The listing builds one solid part. Answer for the finished solid, in the listing's coordinates (mm). Face numbers are marked on the shaded views. A direction names the side the tool comes from. Round coordinates to 2 decimals unless told otherwise and drop trailing zeros. Loops run counter-clockwise (first coordinate to the right, second up) from the corner with the lowest first, then second, coordinate; pieces in that order, holes last. Notation, with made-up numbers: (5, 11.25) - (18, 11.25) arc R31 ccw to (18, 41.25) - close; hole circle Ø11 at (20, 39.5). An arc over 180 degrees is marked (long way). Write item = value, one per line. Start each with the question number.
1) For a pull along Z with two mould halves and no side action, classify the marked faces 1, 2 and 3 as released by +Z, released by -Z, zero draft, split by the parting line, or undercut.
2) Section C-C, the plane y = -14 is taken. Determine the outline of the cut face in (x, z).
3) Section A-A, the plane z = -18.5 is taken. Determine the outline of the cut face in (x, y), and give its area (3 significant figures).
4) Straight lines are drawn through the part: line 1 along X through (y, z) = (-11.5, 36.5); line 2 along Y through (x, z) = (30, 21); line 3 along Z through (x, y) = (-33, 67). For each, find the intervals that lie inside material, in ascending order.
5) Section B-B, the plane x = 20.5 is taken. Determine the outline of the cut face in (y, z).
6) Given pin 1 Ø12.5 at (x, y) = (41.5, -8.5) entering from -Z; pin 2 Ø7.5 at (y, z) = (-9.5, 0.5) entering from -X; pin 3 Ø3 at (x, y) = (-37.5, -51.5) entering from +Z; pin 4 Ø4 at (x, z) = (5, 34) entering from +Y, each flat-ended and moving along its own axis, determine where each tip first touches the part or whether it passes through.
7) A tool of negligible diameter and unlimited length cuts with its end or side. For the marked faces 4, 5 and 6, from which of +Z, -Z, +X, -X, +Y, -Y can it reach the whole face along a straight path? Write none if from no direction.
8) Section D-D, the plane z = 33 is taken. Determine the outline of the cut face in (x, y).
from build123d import *

# Parameters (mm, degrees)
F1_DEPTH      = 25.4
F2_R          = 10.3575918664
F3_DEPTH      = 82.7624946833
F3_DEPTH_BACK = 25.4
F4_DEPTH      = 25.4
F5_DEPTH      = 211.4430963993


with BuildPart() as f1:
    # F0 (on Front) → F1 (new body)
    with BuildSketch(Plane.XZ):
        Polygon((-54.8551306129, 59.1857582331), (-54.8551306129, 13.9228226617), (-29.6127572656, 0), (-29.6127572656, -32.6884873211), (-54.8551306129, -32.6884873211), (-54.8551306129, -56.3453622162), (-17.4506641924, -56.3453622162), (-17.4506641924, 45.9188297391), (8.5172532126, 45.9188297391), (8.5172532126, 16.1184109747), (38.0811914802, 16.1184109747), (38.0811914802, -25.0818282366), (12.4506652355, -25.0818282366), (12.4506652355, -55.7573884726), (52.5093525648, -55.7573884726), (52.5093525648, 59.1857582331), align=None)
    extrude(amount=F1_DEPTH)

    # F2 (on Front) → F3 (join, two sides)
    with BuildSketch(Plane.XZ) as f3_sk:
        with Locations((-28.0219614506, 29.9158245325)):
            Circle(F2_R)
    extrude(amount=-F3_DEPTH)
    extrude(f3_sk.sketch, amount=F3_DEPTH_BACK)

    # F4 (add): a face of the model
    f4_faces = [f1.faces().sort_by_distance(p)[0] for p in [
        (-28.0219614506, 82.7624946833, 29.9158245325),
    ]]
    extrude(f4_faces, amount=F4_DEPTH)

    # F5 (add): a face of the model
    f5_faces = [f1.faces().sort_by_distance(p)[0] for p in [
        (-28.0219614506, 108.1624946833, 29.9158245325),
    ]]
    extrude(f5_faces, amount=-F5_DEPTH)


solid = f1.part
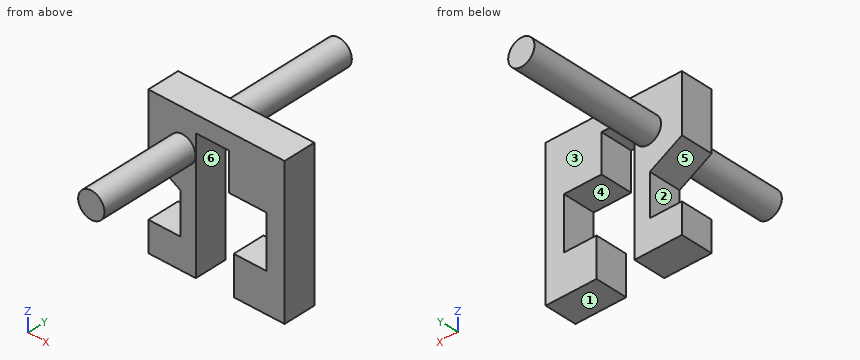
Geometry check:
q1.face_1 = released by -Z
q1.face_2 = undercut
q1.face_3 = zero draft
q2.outline = (-54.86, -56.35) - (-17.45, -56.35) - (-17.45, 45.92) - (8.52, 45.92) - (8.52, 16.12) - (38.08, 16.12) - (38.08, -25.08) - (12.45, -25.08) - (12.45, -55.76) - (52.51, -55.76) - (52.51, 59.19) - (-54.86, 59.19) - (-54.86, 13.92) - (-29.61, 0) - (-29.61, -32.69) - (-54.86, -32.69) - close
q3.outline = (-29.61, -25.4) - (-17.45, -25.4) - (-17.45, 0) - (-29.61, 0) - close; (38.08, -25.4) - (52.51, -25.4) - (52.51, 0) - (38.08, 0) - close
q3.area = 675 mm2
q4.line_1 = -54.86 to -17.45, 8.52 to 52.51
q4.line_2 = -25.4 to 0
q4.line_3 = 20.83 to 39
q5.outline = (-25.4, -55.76) - (0, -55.76) - (0, -25.08) - (-25.4, -25.08) - close; (-25.4, 16.12) - (0, 16.12) - (0, 59.19) - (-25.4, 59.19) - close
q6.pin_1 = -55.76
q6.pin_2 = -37.32
q6.pin_3 = 36.52
q6.pin_4 = through
q7.face_4 = +Y, -Y
q7.face_5 = -X, +Y, -Y
q7.face_6 = -Z, +Y, -Y
q8.outline = (-54.86, -25.4) - (-37.91, -25.4) - (-37.91, -103.28) - (-18.13, -103.28) - (-18.13, -25.4) - (-17.45, -25.4) - (-17.45, 0) - (-18.13, 0) - (-18.13, 108.16) - (-37.91, 108.16) - (-37.91, 0) - (-54.86, 0) - close; (8.52, -25.4) - (52.51, -25.4) - (52.51, 0) - (8.52, 0) - close
